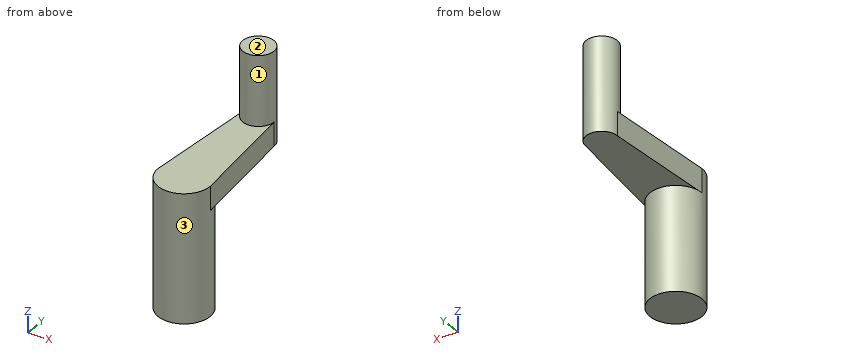
Autodesk Inventor part; units mm, degrees
ref_plane "YZ Plane" through (0, 0, 0) normal (1, 0, 0) x (0, 1, 0)
ref_plane "XZ Plane" through (0, 0, 0) normal (0, 1, 0) x (-1, 0, 0)
ref_plane "XY Plane" through (0, 0, 0) normal (0, 0, 1) x (1, 0, 0)
sketch "Sketch1" plane through (0, 0, 0) normal (0, 0, 1) x (1, 0, 0)
  circle A0 centre (0, 0) radius 12.5
  dimension "d0" = 25
extrude "Extrusion1" add sketch "Sketch1" along normal blind 50
sketch "Sketch2" plane through (0, 0, 50) normal (0, 0, 1) x (1, 0, 0)
  circle A0 centre (0, 55.1215) radius 7.5
  line L0 (-7.5, 55.1215) -> (-12.5, 0)
  circle A1 centre (0, 0) radius 12.5
  line L1 (7.5, 55.1215) -> (12.5, 0)
  dimension "d3" = 15
extrude "Extrusion2" add sketch "Sketch2" along normal blind 11.5 contours L1 A1 L0 A0 | L1 A1 L0
extrude "Extrusion3" add sketch "Sketch2" along normal blind 45 contours A0
Geometry check sheet. Reference: the model listing, model coordinates, mm. Face numbers are marked on the shaded views. A direction names the side the tool comes from. Round coordinates to 2 decimals unless told otherwise and drop trailing zeros. Loops run counter-clockwise (first coordinate to the right, second up) from the corner with the lowest first, then second, coordinate; pieces in that order, holes last.
Item 1: Access from +Z, -Z, +X, -X, +Y, -Y to the whole of each face (thin tool, end or side, straight path). Record for the marked faces 1, 2 and 3.
Item 2: Cross-section at B-B on y = 8. Record the boundary of the cut face in (x, z), then the cut area to 3 significant figures.
Item 3: Cross-section at C-C on z = 48.5. Record the boundary of the cut face in (x, y).
Item 4: Cross-section at A-A on x = 0. Record the boundary of the cut face in (y, z), then the cut area to 3 significant figures.
Item 5: Gauge pin test, flat ends, axial feed: pin 1 (1 mm diameter, centred on x = 3.5, z = 58, fed in from -Y); pin 2 (12.5 mm diameter, centred on x = 4, y = 47, fed in from -Z); pin 3 (1 mm diameter, centred on x = -3.5, y = 9, fed in from +Z). Record the tip position at first contact, or that the pin passes through.
Item 6: Cross-section at D-D on z = 72. Record the boundary of the cut face in (x, y), then the cut area to 3 significant figures.
Item 7: Thickness scan on line 1 (Z direction, x = -2.5, y = 39.5); line 2 (Z direction, x = 2.75, y = -4); line 3 (Y direction, x = -0.5, z = 86.5). Record the ranges inside material, lowest first.
Answer sheet:
1. face 1: +Z
1. face 2: +Z, +X, -X, +Y, -Y
1. face 3: -Z
2. outline: (-11.77, 50) - (-9.6, 50) - (-9.6, 0) - (9.6, 0) - (9.6, 50) - (11.77, 50) - (11.77, 61.5) - (-11.77, 61.5) - close
2. area: 1,230 mm2
3. outline: circle Ø25 at (0, 0)
4. outline: (-12.5, 0) - (12.5, 0) - (12.5, 50) - (62.62, 50) - (62.62, 95) - (47.62, 95) - (47.62, 61.5) - (-12.5, 61.5) - close
4. area: 2,620 mm2
5. pin 1: stops at y = -12.13
5. pin 2: stops at z = 50
5. pin 3: stops at z = 61.5
6. outline: circle Ø15 at (0, 55.12)
6. area: 177 mm2
7. line 1: z = 50 to 61.5
7. line 2: z = 0 to 61.5
7. line 3: y = 47.64 to 62.6
